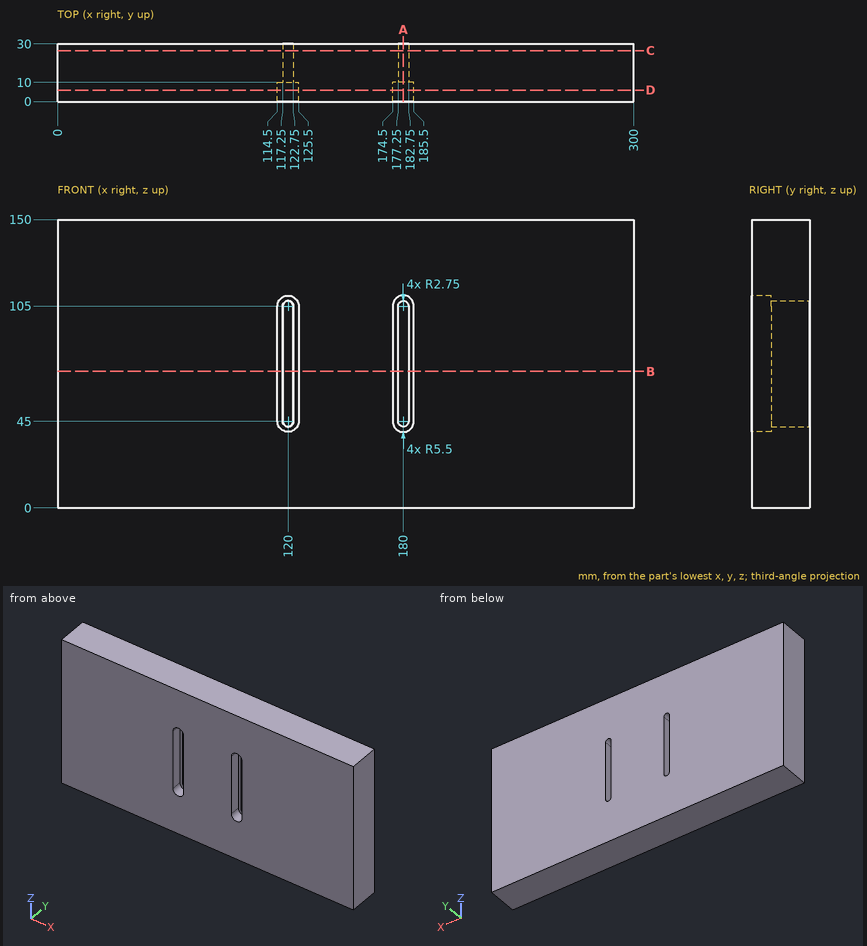
Design review of the part shown in the three views and the two pictorial views. Dimensions are in mm from the part's minimum x, y and z. Give positions to 0.01 mm unless a question says otherwise; leave off trailing zeros. Loops run counter-clockwise (first coordinate to the right, second up) from the corner with the lowest first, then second, coordinate; pieces in that order, holes last. Notation, with made-up numbers: (26, 50.5) - (61, 50.5) arc R36 ccw to (61, 88.5) - close; hole circle Ø8 at (2.25, 88.25). An arc over 180 degrees is marked (long way). Answer as a JSON object with one key per item and string values.
Q1. Add section D-D on y = 6. State the section outline as (x, z) points.
Worked out:
{"outline": "(0, 0) - (300, 0) - (300, 150) - (0, 150) - close; hole (114.5, 45) arc R5.5 ccw to (125.5, 45) - (125.5, 105) arc R5.5 ccw to (114.5, 105) - close; hole (174.5, 45) arc R5.5 ccw to (185.5, 45) - (185.5, 105) arc R5.5 ccw to (174.5, 105) - close"}
Q2. Insertion check: pin 1 (3.5 mm diameter, centred on x = 122.5, z = 68.5, fed in from -Y). The pin has a flat end and moves straight along its axis. Give the tip position at first contact, or say it passes through.
Worked out:
{"pin 1": "stops at y = 10"}
Q3. To check wall thickness, follow line 1 along X through (y, z) = (20, 92.5); line 2 along X through (y, z) = (7, 75). State the ranges of each line that lie inside material, in increasing order.
Worked out:
{"line 1": "x = 0 to 117.25, 122.75 to 177.25, 182.75 to 300", "line 2": "x = 0 to 114.5, 125.5 to 174.5, 185.5 to 300"}
Q4. Add section A-A on x = 180. State the section outline as (y, z) points.
Worked out:
{"outline": "(0, 0) - (30, 0) - (30, 42.25) - (10, 42.25) - (10, 39.5) - (0, 39.5) - close; (0, 110.5) - (10, 110.5) - (10, 107.75) - (30, 107.75) - (30, 150) - (0, 150) - close"}
Q5. Add section C-C on y = 26.5. State the section outline as (x, z) points.
Worked out:
{"outline": "(0, 0) - (300, 0) - (300, 150) - (0, 150) - close; hole (117.25, 45) arc R2.75 ccw to (122.75, 45) - (122.75, 105) arc R2.75 ccw to (117.25, 105) - close; hole (177.25, 45) arc R2.75 ccw to (182.75, 45) - (182.75, 105) arc R2.75 ccw to (177.25, 105) - close"}
Q6. Add section B-B on z = 71. State the section outline as (x, y) points.
Worked out:
{"outline": "(0, 0) - (114.5, 0) - (114.5, 10) - (117.25, 10) - (117.25, 30) - (0, 30) - close; (122.75, 10) - (125.5, 10) - (125.5, 0) - (174.5, 0) - (174.5, 10) - (177.25, 10) - (177.25, 30) - (122.75, 30) - close; (182.75, 10) - (185.5, 10) - (185.5, 0) - (300, 0) - (300, 30) - (182.75, 30) - close"}
